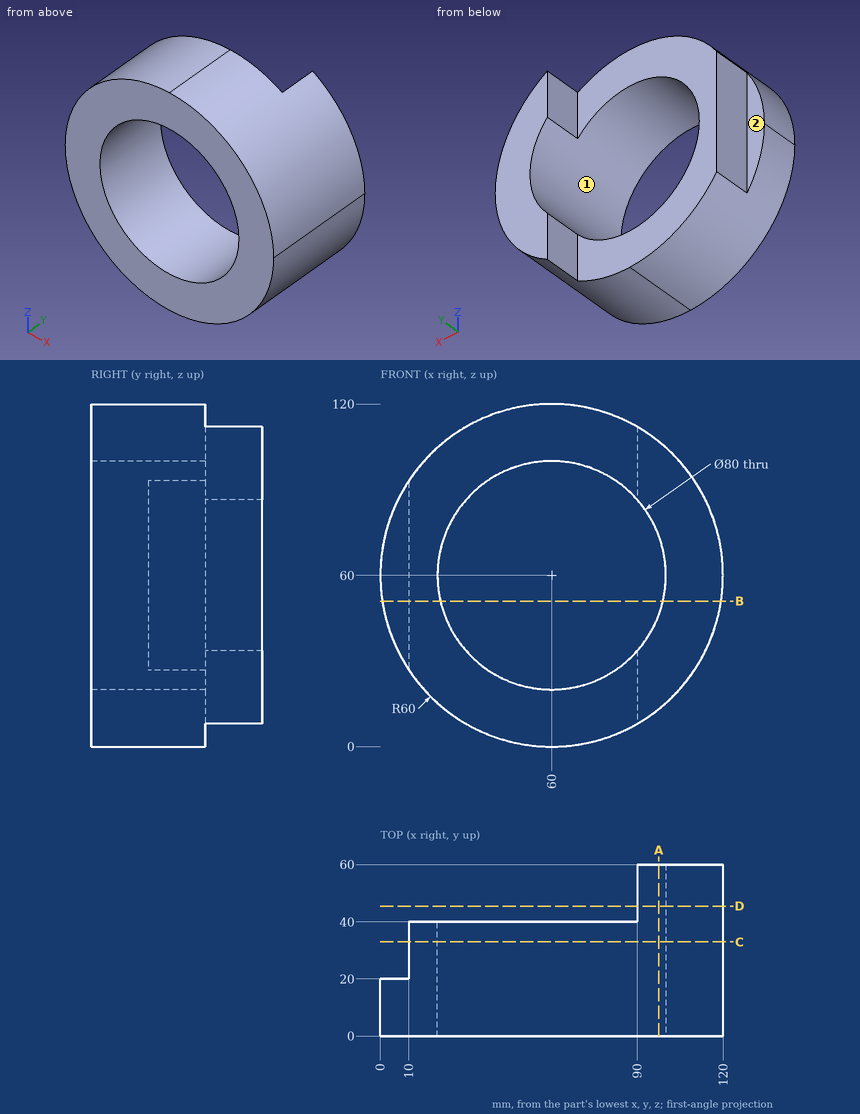
Job drawing, mm, ordinate dimensions from the low corner. One solid piece. A direction names the side the tool comes from. Coordinates: 2 decimals unless noted, no trailing zeros. Order: outer loops, then holes, each group sorted by start corner. A loop starts at its lowest first (then second) coordinate and runs counter-clockwise, first axis right, second up. Notation, with made-up numbers: (3.5, 41) -> (12.5, 41) arc R24 cw to (12.5, 71) -> close; hole circle Ø10 at (6.25, 13). An arc over 180 degrees is marked (long way). Answer in a Markdown table with one row per item. Add a question column.
Q1. Wall check: line 1 along Z through (x, y) = (60, 24); line 2 along X through (y, z) = (25.5, 60). Give the ranges that are in metal, low to high. Write a range as [from, to].
Q2. Drop flat-ended pins along their axis: pin 1 (16 mm diameter, centred on y = 50, z = 19.5, fed in from -X); pin 2 (5 mm diameter, centred on x = 6, z = 45, fed in from +Y); pin 3 (6 mm diameter, centred on y = 18, z = 87.5, fed in from -X); pin 4 (10 mm diameter, centred on x = 16.5, z = 50.5, fed in from -Y). Give the stop position or say it passes through.
Q3. Band-saw the part on B-B, the plane z = 51. List the corners of the cut face in (x, y), then the cut area to 3 significant figures.
Q4. Which spindle directions (+Z, -Z, +X, -X, +Y, -Y) get a long thin tool onto all of the face, cutting with end or side? Do the marked faces 1 and 2. Say none if no direction does.
Q5. Band-saw the part on C-C, the plane y = 33. List the corners of the cut face in (x, z).
Q6. Band-saw the part on A-A, the plane x = 97.5. List the corners of the cut face in (y, z), then the cut area to 3 significant figures.
Q7. Band-saw the part on D-D, the plane y = 45.5. List the corners of the cut face in (x, z).
Answers follow:
| question | item | result |
|---|---|---|
| 1 | line 1 | [0, 20], [100, 120] |
| 1 | line 2 | [10, 20], [100, 120] |
| 2 | pin 1 | x = 90 |
| 2 | pin 2 | y = 20 |
| 2 | pin 3 | x = 5.23 |
| 2 | pin 4 | y = 0 |
| 3 | outline | (0.68, 0) -> (21.03, 0) -> (21.03, 40) -> (10, 40) -> (10, 20) -> (0.68, 20) -> close; (98.97, 0) -> (119.32, 0) -> (119.32, 60) -> (98.97, 60) -> close |
| 3 | area | 1,850 mm^2 |
| 4 | face 1 | +Y, -Y |
| 4 | face 2 | +Z, -Z, -X, +Y |
| 5 | outline | (10, 26.83) arc R60 ccw (long way) to (10, 93.17) -> close; hole circle Ø80 at (60, 60) |
| 6 | outline | (0, 13.16) -> (60, 13.16) -> (60, 46.08) -> (0, 46.08) -> close; (0, 73.92) -> (60, 73.92) -> (60, 106.84) -> (0, 106.84) -> close |
| 6 | area | 3,950 mm^2 |
| 7 | outline | (90, 8.04) arc R60 ccw to (90, 111.96) -> (90, 86.46) arc R40 cw to (90, 33.54) -> close |
